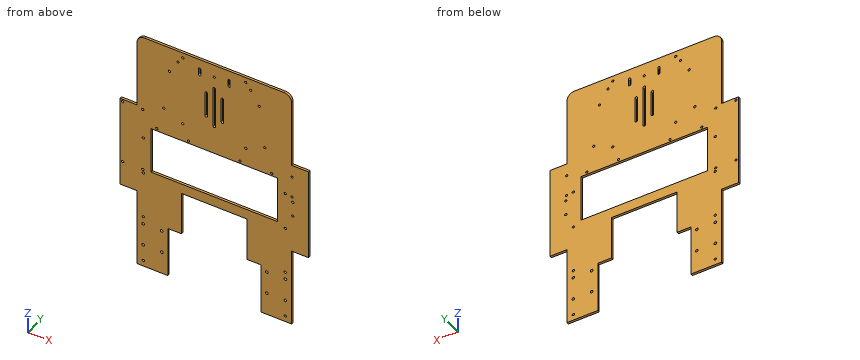
```python
from build123d import *

# Parameters (mm, degrees)
SKETCH_1_W           = 200
SKETCH_1_H           = 375
EXTRUDE_1_DEPTH      = 3
SKETCH_2_R           = 1.75
CUT_EXTRUDE_1_DEPTH  = 10
SKETCH_3_R           = 1.5
CUT_EXTRUDE_2_DEPTH  = 10
SKETCH_4_R           = 1.5
CUT_EXTRUDE_3_DEPTH  = 10
SKETCH_5_W           = 210
SKETCH_5_H           = 50.72585274
CUT_EXTRUDE_5_DEPTH  = 34.39
SKETCH_8_R           = 1.5
EXTRUDE_2_DEPTH      = 3
SKETCH_9_W           = 163.883016164
SKETCH_9_H           = 75
CUT_EXTRUDE_6_DEPTH  = 10
CUT_EXTRUDE_7_DEPTH  = 3
SKETCH_11_R          = 1.5
CUT_EXTRUDE_8_DEPTH  = 6
SKETCH_12_R          = 1.5
CUT_EXTRUDE_9_DEPTH  = 3
CUT_EXTRUDE_10_DEPTH = 163.8
SKETCH_16_W          = 173.87129554
SKETCH_16_H          = 50.701400684
EXTRUDE_4_DEPTH      = 3
SKETCH_18_W          = 121.748470969
SKETCH_18_H          = 3
EXTRUDE_5_DEPTH      = 22
SKETCH_19_W          = 17.27862471
SKETCH_19_H          = 21.556396233
CUT_EXTRUDE_11_DEPTH = 22
SKETCH_20_R          = 1.5
CUT_EXTRUDE_12_DEPTH = 5
SKETCH_21_R          = 1.5
CUT_EXTRUDE_13_DEPTH = 6
SKETCH_22_W          = 163.883016164
SKETCH_22_H          = 4.895548477
EXTRUDE_6_DEPTH      = 3
CUT_EXTRUDE_14_DEPTH = 10
CUT_EXTRUDE_15_DEPTH = 10
SKETCH_25_R          = 1.5
CUT_EXTRUDE_16_DEPTH = 5
SKETCH_26_R          = 1.5
CUT_EXTRUDE_17_DEPTH = 10
SKETCH_27_R          = 1.5
CUT_EXTRUDE_18_DEPTH = 3
SKETCH_28_R          = 1.5
CUT_EXTRUDE_19_DEPTH = 3
FILLET_1_R           = 10


with BuildPart() as part:
    # 草图1 → 凸台-拉伸1 (new body)
    with BuildSketch(Plane(origin=(0, 0, 0), x_dir=(1, 0, 0), z_dir=(0, 1, 0))):
        Rectangle(SKETCH_1_W, SKETCH_1_H)
    extrude(amount=EXTRUDE_1_DEPTH)

    # 草图2 → 切除-拉伸1 (cut)
    with BuildSketch(Plane.XZ):
        with Locations(Location((-68, -157.5, 0), (0, 0, 270))):
            Circle(SKETCH_2_R)
        with Locations(Location((-92, -157.5, 0), (0, 0, 270))):
            Circle(SKETCH_2_R)
        with Locations(Location((-92, -127.5, 0), (0, 0, 270))):
            Circle(SKETCH_2_R)
        with Locations(Location((-68, -127.5, 0), (0, 0, 270))):
            Circle(SKETCH_2_R)
        with Locations(Location((68, -157.5, 0), (0, 0, 270))):
            Circle(SKETCH_2_R)
        with Locations(Location((92, -157.5, 0), (0, 0, 270))):
            Circle(SKETCH_2_R)
        with Locations(Location((92, -127.5, 0), (0, 0, 270))):
            Circle(SKETCH_2_R)
        with Locations(Location((68, -127.5, 0), (0, 0, 270))):
            Circle(SKETCH_2_R)
    extrude(amount=-CUT_EXTRUDE_1_DEPTH, mode=Mode.SUBTRACT)

    # 草图3 → 切除-拉伸2 (cut)
    with BuildSketch(Plane(origin=(0, 3, 0), x_dir=(1, 0, 0), z_dir=(0, 1, 0))):
        with Locations(Location((0, -119.896683452, 0), (0, 0, 270))):
            Circle(SKETCH_3_R)
    extrude(amount=-CUT_EXTRUDE_2_DEPTH, mode=Mode.SUBTRACT)

    # 草图4 → 切除-拉伸3 (cut)
    with BuildSketch(Plane(origin=(0, 3, 0), x_dir=(1, 0, 0), z_dir=(0, 1, 0))):
        with Locations(Location((19, -119.896683452, 0), (0, 0, 270))):
            Circle(SKETCH_4_R)
        with Locations(Location((-19, -119.896683452, 0), (0, 0, 270))):
            Circle(SKETCH_4_R)
    extrude(amount=-CUT_EXTRUDE_3_DEPTH, mode=Mode.SUBTRACT)

    # 草图5 → 切除-拉伸5 (cut)
    with BuildSketch(Plane.XZ):
        with Locations((0, 162.13707363)):
            Rectangle(SKETCH_5_W, SKETCH_5_H)
    extrude(amount=-CUT_EXTRUDE_5_DEPTH, mode=Mode.SUBTRACT)

    # 草图8 → 凸台-拉伸2 (add)
    with BuildSketch(Plane.ZY.offset(100)):
        with BuildLine():
            Line((34.419687156, 14.367900616), (37.872189, 3))
            Line((37.872189, 3), (25.226116951, 3))
            Line((25.226116951, 3), (28.678618796, 14.367900616))
            ThreePointArc((28.678618796, 14.367900616), (31.549152976, 16.496101602), (34.419687156, 14.367900616))
        make_face()
        with Locations((31.549152976, 13.496101602)):
            Circle(SKETCH_8_R, mode=Mode.SUBTRACT)
    extrude(amount=-EXTRUDE_2_DEPTH)

    # 草图9 → 切除-拉伸6 (cut)
    with BuildSketch(Plane.XZ):
        with Locations((0, 18.152093794)):
            Rectangle(SKETCH_9_W, SKETCH_9_H)
    extrude(amount=-CUT_EXTRUDE_6_DEPTH, mode=Mode.SUBTRACT)

    # 草图10 → 切除-拉伸7 (cut)
    with BuildSketch(Plane.XZ):
        Polygon((-60.157077223, -120.5533384), (-42.238826625, -120.5533384), (-42.238826625, -63.289088645), (42.238826625, -63.289088645), (42.238826625, -120.5533384), (60.157077223, -120.5533384), (60.157077223, -187.5), (-60.157077223, -187.5), align=None)
    extrude(amount=-CUT_EXTRUDE_7_DEPTH, mode=Mode.SUBTRACT)

    # 草图11 → 切除-拉伸8 (cut)
    with BuildSketch(Plane(origin=(0, 3, 0), x_dir=(1, 0, 0), z_dir=(0, 1, 0))):
        with Locations(Location((-91.756220162, 179.630143817, 0), (0, 0, 270))):
            Circle(SKETCH_11_R)
        with Locations(Location((-91.756220162, 117.5, 0), (0, 0, 270))):
            Circle(SKETCH_11_R)
        with Locations(Location((-91.756220162, 55.369856183, 0), (0, 0, 270))):
            Circle(SKETCH_11_R)
        with Locations(Location((91.756220162, 55.369856183, 0), (0, 0, 270))):
            Circle(SKETCH_11_R)
        with Locations(Location((91.756220162, 117.5, 0), (0, 0, 270))):
            Circle(SKETCH_11_R)
        with Locations(Location((91.756220162, 179.630143817, 0), (0, 0, 270))):
            Circle(SKETCH_11_R)
    extrude(amount=-CUT_EXTRUDE_8_DEPTH, mode=Mode.SUBTRACT)

    # 草图12 → 切除-拉伸9 (cut)
    with BuildSketch(Plane(origin=(0, 3, 0), x_dir=(1, 0, 0), z_dir=(0, 1, 0))):
        with Locations(Location((-91.756220162, 5.808361465, 0), (0, 0, 270))):
            Circle(SKETCH_12_R)
        with Locations(Location((91.756220162, 5.808361465, 0), (0, 0, 270))):
            Circle(SKETCH_12_R)
    extrude(amount=-CUT_EXTRUDE_9_DEPTH, mode=Mode.SUBTRACT)

    # 草图14 → 切除-拉伸10 (cut)
    with BuildSketch(Plane(origin=(0, 3, 0), x_dir=(1, 0, 0), z_dir=(0, 1, 0))):
        Polygon((81.941508082, 19.347906206), (81.941508082, 49.288971574), (81.941508082, 54.851401937), (-81.941508082, 54.851401937), (-81.941508082, 49.288971574), (-81.941508082, 19.347906206), align=None)
    extrude(amount=-CUT_EXTRUDE_10_DEPTH, mode=Mode.SUBTRACT)

    # 草图16 → 凸台-拉伸4 (add)
    with BuildSketch(Plane(origin=(0, 3, 0), x_dir=(1, 0, 0), z_dir=(0, 1, 0))):
        with Locations((0.567640728, -37.155553542)):
            Rectangle(SKETCH_16_W, SKETCH_16_H)
    extrude(amount=-EXTRUDE_4_DEPTH)

    # 草图18 → 凸台-拉伸5 (add)
    with BuildSketch(Plane.ZY.offset(100)):
        with Locations((-23.168262452, 1.5)):
            Rectangle(SKETCH_18_W, SKETCH_18_H)
    extrude_5 = extrude(amount=EXTRUDE_5_DEPTH)

    # 草图19 → 切除-拉伸11 (cut)
    with BuildSketch(Plane.ZY.offset(100)):
        with Locations((31.606580178, 13.778198117)):
            Rectangle(SKETCH_19_W, SKETCH_19_H)
    extrude(amount=-CUT_EXTRUDE_11_DEPTH, mode=Mode.SUBTRACT)

    # 镜向1: 凸台-拉伸5 across plane
    add(extrude_5.mirror(Plane(origin=(0, 0, 0), x_dir=(0, 0, 1), z_dir=(1, 0, 0))))

    # 草图20 → 切除-拉伸12 (cut)
    with BuildSketch(Plane.XZ):
        with Locations(Location((-92.437313721, 34.301588012, 0), (0, 0, 270))):
            Circle(SKETCH_20_R)
        with Locations(Location((-118.512686279, 34.301588012, 0), (0, 0, 270))):
            Circle(SKETCH_20_R)
        with Locations(Location((-92.437313721, -50.669641947, 0), (0, 0, 270))):
            Circle(SKETCH_20_R)
        with Locations(Location((-118.512686279, -50.669641947, 0), (0, 0, 270))):
            Circle(SKETCH_20_R)
    extrude(amount=-CUT_EXTRUDE_12_DEPTH, mode=Mode.SUBTRACT)

    # 草图21 → 切除-拉伸13 (cut)
    with BuildSketch(Plane(origin=(0, 3, 0), x_dir=(1, 0, 0), z_dir=(0, 1, 0))):
        with Locations(Location((101.493568208, 33.673307051, 0), (0, 0, 270))):
            Circle(SKETCH_21_R)
        with Locations(Location((101.493568208, 14.236029002, 0), (0, 0, 270))):
            Circle(SKETCH_21_R)
        with Locations(Location((100.46791463, -21.089263072, 0), (0, 0, 270))):
            Circle(SKETCH_21_R)
        with Locations(Location((100.46791463, 6.938433331, 0), (0, 0, 270))):
            Circle(SKETCH_21_R)
    extrude(amount=-CUT_EXTRUDE_13_DEPTH, mode=Mode.SUBTRACT)

    # 草图22 → 凸台-拉伸6 (add)
    with BuildSketch(Plane(origin=(0, 3, 0), x_dir=(1, 0, 0), z_dir=(0, 1, 0))):
        with Locations((0, 52.403627699)):
            Rectangle(SKETCH_22_W, SKETCH_22_H)
    extrude(amount=-EXTRUDE_6_DEPTH)

    # 草图23 → 切除-拉伸14 (cut)
    with BuildSketch(Plane.XZ):
        with BuildLine():
            Line((-12.1, 93.046379783), (-12.1, 60.426325499))
            ThreePointArc((-12.1, 60.426325499), (-10.5, 58.826325499), (-8.9, 60.426325499))
            Line((-8.9, 60.426325499), (-8.9, 93.046379783))
            ThreePointArc((-8.9, 93.046379783), (-10.5, 94.646379783), (-12.1, 93.046379783))
        make_face()
        with BuildLine():
            Line((8.9, 93.046379783), (8.9, 60.426325499))
            ThreePointArc((8.9, 60.426325499), (10.5, 58.826325499), (12.1, 60.426325499))
            Line((12.1, 60.426325499), (12.1, 93.046379783))
            ThreePointArc((12.1, 93.046379783), (10.5, 94.646379783), (8.9, 93.046379783))
        make_face()
        with BuildLine():
            Line((-1.6, 103.546379783), (-1.6, 49.926325499))
            ThreePointArc((-1.6, 49.926325499), (0, 48.326325499), (1.6, 49.926325499))
            Line((1.6, 49.926325499), (1.6, 103.546379783))
            ThreePointArc((1.6, 103.546379783), (0, 105.146379783), (-1.6, 103.546379783))
        make_face()
    extrude(amount=-CUT_EXTRUDE_14_DEPTH, mode=Mode.SUBTRACT)

    # 草图24 → 切除-拉伸15 (cut)
    with BuildSketch(Plane(origin=(0, 3, 0), x_dir=(1, 0, 0), z_dir=(0, 1, 0))):
        with BuildLine():
            Line((-20.5, -115.409589276), (-20.5, -119.896683452))
            Line((-20.5, -119.896683452), (-20.5, -123.292696741))
            ThreePointArc((-20.5, -123.292696741), (-19, -124.792696741), (-17.5, -123.292696741))
            Line((-17.5, -123.292696741), (-17.5, -119.896683452))
            Line((-17.5, -119.896683452), (-17.5, -115.409589276))
            Line((-17.5, -115.409589276), (-17.5, -115.10448085))
            ThreePointArc((-17.5, -115.10448085), (-19, -113.749297424), (-20.5, -115.10448085))
            Line((-20.5, -115.10448085), (-20.5, -115.409589276))
        make_face()
        with BuildLine():
            ThreePointArc((17.5, -123.292696741), (19, -124.792696741), (20.5, -123.292696741))
            Line((20.5, -123.292696741), (20.5, -119.896683452))
            Line((20.5, -119.896683452), (20.5, -115.409589276))
            Line((20.5, -115.409589276), (20.5, -115.10448085))
            ThreePointArc((20.5, -115.10448085), (19, -113.749297424), (17.5, -115.10448085))
            Line((17.5, -115.10448085), (17.5, -115.409589276))
            Line((17.5, -115.409589276), (17.5, -119.896683452))
            Line((17.5, -119.896683452), (17.5, -123.292696741))
        make_face()
    extrude(amount=-CUT_EXTRUDE_15_DEPTH, mode=Mode.SUBTRACT)

    # 草图25 → 切除-拉伸16 (cut)
    with BuildSketch(Plane(origin=(0, 3, 0), x_dir=(1, 0, 0), z_dir=(0, 1, 0))):
        with Locations(Location((-74.307985478, -15.126608199, 0), (0, 0, 270))):
            Circle(SKETCH_25_R)
        with Locations(Location((-33.249974851, -15.126608199, 0), (0, 0, 270))):
            Circle(SKETCH_25_R)
        with Locations(Location((33.249974851, -15.126608199, 0), (0, 0, 270))):
            Circle(SKETCH_25_R)
        with Locations(Location((74.307985478, -15.126608199, 0), (0, 0, 270))):
            Circle(SKETCH_25_R)
    extrude(amount=-CUT_EXTRUDE_16_DEPTH, mode=Mode.SUBTRACT)

    # 草图26 → 切除-拉伸17 (cut)
    with BuildSketch(Plane(origin=(0, 3, 0), x_dir=(1, 0, 0), z_dir=(0, 1, 0))):
        with Locations(Location((-65.342005187, -47.889665829, 0), (0, 0, 270))):
            Circle(SKETCH_26_R)
        with Locations(Location((65.342005187, -47.889665829, 0), (0, 0, 270))):
            Circle(SKETCH_26_R)
        with Locations(Location((46.986453842, -121.386909585, 0), (0, 0, 270))):
            Circle(SKETCH_26_R)
        with Locations(Location((-46.986453842, -121.386909585, 0), (0, 0, 270))):
            Circle(SKETCH_26_R)
    extrude(amount=-CUT_EXTRUDE_17_DEPTH, mode=Mode.SUBTRACT)

    # 草图27 → 切除-拉伸18 (cut)
    with BuildSketch(Plane(origin=(0, 3, 0), x_dir=(1, 0, 0), z_dir=(0, 1, 0))):
        with Locations(Location((-40.75, -36.322032373, 0), (0, 0, 270))):
            Circle(SKETCH_27_R)
        with Locations(Location((40.75, -36.322032373, 0), (0, 0, 270))):
            Circle(SKETCH_27_R)
        with Locations(Location((40.75, -129.822032373, 0), (0, 0, 270))):
            Circle(SKETCH_27_R)
        with Locations(Location((-40.75, -129.822032373, 0), (0, 0, 270))):
            Circle(SKETCH_27_R)
    extrude(amount=-CUT_EXTRUDE_18_DEPTH, mode=Mode.SUBTRACT)

    # 草图28 → 切除-拉伸19 (cut)
    with BuildSketch(Plane(origin=(0, 3, 0), x_dir=(1, 0, 0), z_dir=(0, 1, 0))):
        with Locations(Location((-58.033655971, -103.347880676, 0), (0, 0, 270))):
            Circle(SKETCH_28_R)
        with Locations(Location((58.033655971, -103.347880676, 0), (0, 0, 270))):
            Circle(SKETCH_28_R)
    extrude(amount=-CUT_EXTRUDE_19_DEPTH, mode=Mode.SUBTRACT)

    # 圆角1
    fillet_1_edges = [part.edges().sort_by_distance(p)[0] for p in [
        (100, 1.5, 136.77414726),
        (-100, 1.5, 136.77414726),
    ]]
    fillet(fillet_1_edges, radius=FILLET_1_R)


solid = part.part
```
For this review, take the finished solid that the model builds, in its own axes (mm). Round coordinates to 2 decimals unless told otherwise and drop trailing zeros. Loops run counter-clockwise (first coordinate to the right, second up) from the corner with the lowest first, then second, coordinate; pieces in that order, holes last.
Q1. Add section A-A on z = -109. Write out the cut boundary in (x, y), plus the area to 3 significant figures.
Result sheet:
outline: (-100, 0) - (-42.24, 0) - (-42.24, 3) - (-100, 3) - close; (42.24, 0) - (100, 0) - (100, 3) - (42.24, 3) - close
area: 347 mm2
Q2. Add section C-C on y = 1.5. Give the number of separate pieces and of enclosed holes in the cut face, plus the area to 3 significant figures.
Result sheet:
separate pieces: 1
enclosed holes: 45
area: 46,400 mm2
Q3. Insertion check: pin 1 Ø0.9 at (y, z) = (1, 79) entering from -X; pin 2 Ø2.5 at (x, z) = (91.76, -117.5) entering from +Y; pin 3 Ø1.5 at (x, y) = (-28.5, 0.5) entering from -Z. Each pin has a flat end and moves straight along its axis. Give the tip position at first contact, or say it passes through.
Result sheet:
pin 1: stops at x = -100
pin 2: passes through
pin 3: stops at z = -63.29
Q4. Add section B-B on x = 25.5. Write out the cut boundary in (y, z), plus the area to 3 significant figures.
Result sheet:
outline: (0, -63.29) - (3, -63.29) - (3, -49.96) - (0, -49.96) - close; (0, 11.8) - (3, 11.8) - (3, 136.77) - (0, 136.77) - close
area: 415 mm2
Q5. To check wall thickness, follow line 1 along X through (y, z) = (1, -127.5); line 2 along X through (y, z) = (2.15, 62); line 3 along Z through (x, y) = (51, 1.9). State the ranges of each line that lie inside material, in increasing order.
Result sheet:
line 1: x = -100 to -93.75, -90.25 to -69.75, -66.25 to -60.16, 60.16 to 66.25, 69.75 to 90.25, 93.75 to 100
line 2: x = -100 to -12.1, -8.9 to -1.6, 1.6 to 8.9, 12.1 to 100
line 3: z = -120.55 to -49.96, 11.8 to 136.77
